from build123d import *

# Parameters (mm, degrees)
CYLINDER007_R           = 6
CYLINDER007_DEPTH       = 236
CYLINDER007_PITCH_ANGLE = 90
CYLINDER005_R           = 8
CYLINDER005_DEPTH       = 18
CYLINDER005_PITCH_ANGLE = 90


with BuildPart() as connector_bore:
    # Cylinder007 → Cylinder007 (new body)
    with BuildSketch(Plane.XY):
        Circle(CYLINDER007_R)
    extrude(amount=CYLINDER007_DEPTH)


with BuildPart() as connector_bore_1:
    # Cylinder007 pitch: moved
    add(connector_bore.part.rotate(Axis((0, 0, 0), (0, 1, 0)), CYLINDER007_PITCH_ANGLE))


with BuildPart() as connector_bore_2:
    # Cylinder007 placement: moved
    add(connector_bore_1.part.moved(Location((-45, 0, 0))))


with BuildPart() as cut003:
    # Cylinder005 → Cylinder005 (new body)
    with BuildSketch(Plane.XY):
        Circle(CYLINDER005_R)
    extrude(amount=CYLINDER005_DEPTH)


with BuildPart() as cut003_1:
    # Cylinder005 pitch: moved
    add(cut003.part.rotate(Axis((0, 0, 0), (0, 1, 0)), CYLINDER005_PITCH_ANGLE))


with BuildPart() as cut003_2:
    # Cylinder005 placement: moved
    add(cut003_1.part.moved(Location((163, 0, 0))))

    # Cut003: cut connector_bore
    add(connector_bore_2.part, mode=Mode.SUBTRACT)


solid = cut003_2.part
The model under review builds one solid part; all positions refer to its coordinate system, in mm. Round coordinates to 2 decimals unless told otherwise and drop trailing zeros. Write each loop counter-clockwise with the first axis right and the second up, starting at its lowest first coordinate (ties: lowest second). Pieces come first, ordered by that corner, then holes. Notation, with made-up numbers: (65.5, -24) - (108.5, -24) arc R28 ccw to (108.5, 3) - close; hole circle Ø11 at (-7, 25). An arc over 180 degrees is marked (long way). One line per item, written item: value. Start each with the question number.
1. The part is to be moulded in two halves that separate along Z. For faces 1 (the face through (163, 6, 2)), 2 (the face through (171.874, 1.802, -5.723)), 3 (the face through (171.87, -7.81, 1.73)), say which applies: released by +Z, released by -Z, zero draft, split by the parting line, or undercut.
2. Consider section A-A on y = 0. Write out the cut boundary in (x, z).
3. Clearance check with flat-ended pins moving along their axes: P1, Ø3, axis at x = 168, y = -4.5, coming from the +Z side; P2, Ø3, axis at x = 170, z = 4.5, coming from the +Y side; P3, Ø3, axis at x = 175, y = 4, coming from the -Z side. State where each tip first meets the part, or that it passes through.
4. Consider section D-D on z = 6.25. Write out the cut boundary in (x, y).
5. To check wall thickness, follow L1, parallel to Y at x = 168.5, z = 0; L2, parallel to Y at x = 164.25, z = -3.75; L3, parallel to Z at x = 178, y = -5.5. State the ranges of each line that lie inside material, in increasing order. Write a range as from..to.
6. Consider section C-C on x = 175.25. Write out the cut boundary in (y, z).
Checks:
1. face 1: zero draft
1. face 2: undercut
1. face 3: split by the parting line
2. outline: (163, -8) - (181, -8) - (181, -6) - (163, -6) - close; (163, 6) - (181, 6) - (181, 8) - (163, 8) - close
3. P1: stops at z = 7.42
3. P2: stops at y = 7.42
3. P3: stops at z = -7.6
4. outline: (163, -4.99) - (181, -4.99) - (181, 4.99) - (163, 4.99) - close
5. L1: y = -8..-6, 6..8
5. L2: y = -7.07..-4.68, 4.68..7.07
5. L3: z = -5.81..-2.4, 2.4..5.81
6. outline: circle Ø16 at (0, 0); hole circle Ø12 at (0, 0)
